Verification items for the finished model (mm, model axes). Coordinates: 2 decimals unless noted, no trailing zeros. Order: outer loops, then holes, each group sorted by start corner. A loop starts at its lowest first (then second) coordinate and runs counter-clockwise, first axis right, second up.
Q1. Depth check by flat-ended pin: P1, Ø0.5, axis at x = 0.5, y = 28.5, coming from the -Z side; P2, Ø3.5, axis at y = 0, z = 12.7, coming from the -X side. Enter the tip coordinate at first touch or a pass-through.
Q2. Cross-section at C-C, the plane z = 25.4. Record the boundary of the cut face in (x, y), and give its area (3 significant figures).
Q3. Thickness scan on line 1 (Z direction, x = 1.2, y = 0); line 2 (Y direction, x = 1.55, z = 64.5); line 3 (Y direction, x = 1.2, z = 14.5). Record the ranges inside material, lowest first.
Q4. Draft check along Y on faces 1 (the flat face through (1.588, 4, 40)), 2 (the cylindrical face through (0.783, 27.743, 61.658)), 3 (the cylindrical face through (0.78, 1.12, -6.25)). Enter one of: pulls with the +Y half, pulls with the -Y half, needs draft (parallel to the pull), parting line crosses it, or undercut.
Q5. Cross-section at A-A, the plane x = 0.25. Record the boundary of the cut face in (y, z) (1 decimal), and give its area (3 significant figures).
Q6. Cross-section at B-B, the plane z = 0. Record the boundary of the cut face in (x, y).
Q7. Cross-section at D-D, the plane y = 13. Record the boundary of the cut face in (x, z).
Autodesk Inventor part; units mm, degrees
ref_plane "YZ Plane" through (0, 0, 0) normal (1, 0, 0) x (0, 1, 0)
ref_plane "XZ Plane" through (0, 0, 0) normal (0, 1, 0) x (-1, 0, 0)
ref_plane "XY Plane" through (0, 0, 0) normal (0, 0, 1) x (1, 0, 0)
sketch "main" plane through (0, 0, 0) normal (0, 0, 1) x (1, 0, 0)
  circle A0 centre (10.9635, 21.0817) radius 2.1
  circle A1 centre (10.9635, 21.0817) radius 2.0955
  arc A2 (31.3634, 3.4082) -> (38.0738, 11.3874) centre (-11.9899, 46.6796) ccw
  arc A3 (38.0738, 11.3874) -> (38.1719, 14.8984) centre (35.4788, 13.2167) ccw
  circle A4 centre (10.9635, 46.4817) radius 2.0955
  arc A5 (16.3496, 49.845) -> (4.7897, 47.9673) centre (10.9635, 46.4817) ccw
  line L0 (38.1719, 14.8984) -> (16.3496, 49.845)
  arc A6 (-25.4047, -28.8165) -> (-8.6396, -36.6705) centre (-15.6049, -29.7183) ccw
  line L1 (-8.6396, -36.6705) -> (31.3634, 3.4082)
  line L2 (-25.4047, -28.8165) -> (-24.2459, -16.2232)
  circle A7 centre (10.9635, 33.7817) radius 2.0955
  circle A8 centre (-15.6049, -17.0183) radius 2.1844
  arc A9 (-22.5138, -11.768) -> (-24.2459, -16.2232) centre (-15.6049, -17.0183) ccw
  line L3 (4.7897, 47.9673) -> (-8.9994, -9.3358)
  line L4 (-22.5138, -11.768) -> (-12.0863, -11.768)
  arc A10 (-12.0863, -11.768) -> (-8.9994, -9.3358) centre (-12.0863, -8.593) ccw
  point P0 (5.2874, 13.8034)
  point P1 (39.2673, 13.1442)
  dimension "d0" = 4.191
  dimension "d1" = 4.191
  dimension "d3" = 3.175
  dimension "d4" = 4.191
  dimension "d11" = 3.175
sketch "Sketch1" plane through (0, 0, 0) normal (1, 0, 0) x (0, 1, 0)
  circle A0 centre (0, 25.4) radius 2.1
  circle A1 centre (0, 25.4) radius 2.0955
  arc A2 (-20.3999, 43.0735) -> (-27.1104, 35.0943) centre (22.9534, -0.1979) ccw
  arc A3 (-27.1104, 35.0943) -> (-27.2084, 31.5833) centre (-24.5154, 33.265) ccw
  circle A4 centre (0, 0) radius 2.0955
  arc A5 (-5.3861, -3.3633) -> (6.1738, -1.4856) centre (0, 0) ccw
  line L0 (-27.2084, 31.5833) -> (-5.3861, -3.3633)
  arc A6 (36.3681, 75.2982) -> (19.603, 83.1522) centre (26.5684, 76.2) ccw
  line L1 (19.603, 83.1522) -> (-20.3999, 43.0735)
  line L2 (36.3681, 75.2982) -> (35.2093, 62.7049)
  circle A7 centre (0, 12.7) radius 2.0955
  circle A8 centre (26.5684, 63.5) radius 2.1844
  arc A9 (33.4773, 58.2497) -> (35.2093, 62.7049) centre (26.5684, 63.5) ccw
  line L3 (6.1738, -1.4856) -> (19.9628, 55.8175)
  line L4 (33.4773, 58.2497) -> (23.0497, 58.2497)
  arc A10 (23.0497, 58.2497) -> (19.9628, 55.8175) centre (23.0497, 55.0747) ccw
  point P0 (0, 0)
extrude "Extrusion1" add sketch "Sketch1" along normal blind 1.5875 contours L1 A6 L2 A9 L4 A10 L3 A5 L0 A3 A2
properties part number "sled" material "Acetal Resin, White"
Check values:
1. P1: stops at z = 58.25
1. P2: passes through
2. outline: (0, -23.35) - (1.59, -23.35) - (1.59, -2.1) - (0, -2.1) - close; (0, 2.1) - (1.59, 2.1) - (1.59, 12.64) - (0, 12.64) - close
2. area: 50.5 mm2
3. line 1: z = -6.35 to -2.1, 2.1 to 10.6, 14.8 to 23.3, 27.5 to 63.51
3. line 2: y = 0.99 to 24.63, 28.51 to 35.37
3. line 3: y = -16.54 to -1.07, 1.07 to 10.02
4. face 1: needs draft
4. face 2: undercut
4. face 3: parting line crosses it
5. outline: (-27.2, 31.6) - (-5.4, -3.4) arc R6.4 ccw to (6.2, -1.5) - (20, 55.8) arc R3.2 cw to (23, 58.2) - (33.5, 58.2) arc R8.7 ccw to (35.2, 62.7) - (36.4, 75.3) arc R9.8 ccw to (19.6, 83.2) - (-20.4, 43.1) arc R61.3 ccw to (-27.1, 35.1) arc R3.2 ccw to start; hole circle Ø4.2 at (0, 0); hole circle Ø4.2 at (0, 12.7); hole circle Ø4.2 at (0, 25.4); hole circle Ø4.4 at (26.6, 63.5)
5. area: 2,560 mm2
6. outline: (0, -7.49) - (1.59, -7.49) - (1.59, -2.1) - (0, -2.1) - close; (0, 2.1) - (1.59, 2.1) - (1.59, 6.53) - (0, 6.53) - close
7. outline: (0, 26.88) - (1.59, 26.88) - (1.59, 76.54) - (0, 76.54) - close
